Geometry check sheet. Reference: drawing and pictorial views, mm from the part's lowest x, y, z. Round coordinates to 2 decimals unless told otherwise and drop trailing zeros. Loops run counter-clockwise (first coordinate to the right, second up) from the corner with the lowest first, then second, coordinate; pieces in that order, holes last. Notation, with made-up numbers: (-33.75, -22) -> (-19.75, -22) arc R22 cw to (-19.75, -13) -> close; hole circle Ø10 at (86.5, -14). An arc over 180 degrees is marked (long way). Write item = value, one per line.
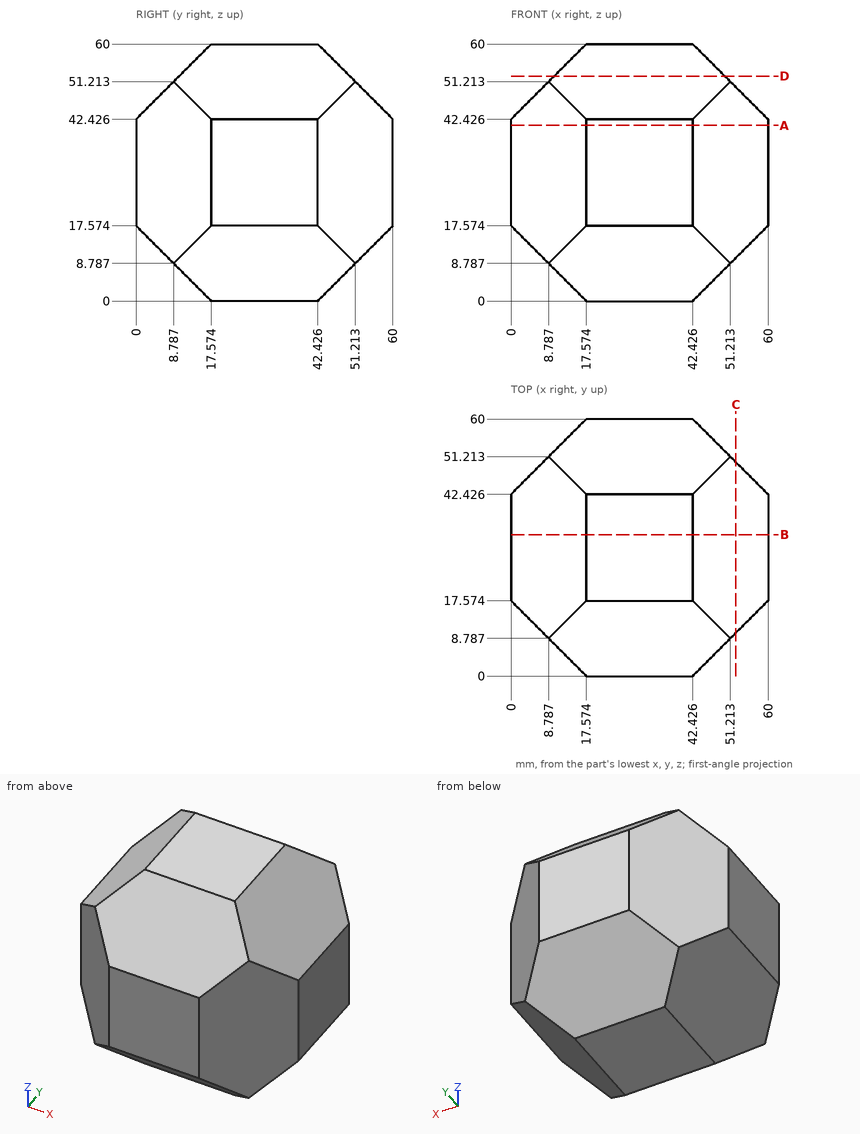
(1) Material ranges on probe 1 along Z at (x, y) = (42.5, 3) (1 decimal); probe 2 along Z at (x, y) = (10.5, 16) (1 decimal); probe 3 along Y at (x, z) = (37, 13.5) (1 decimal), recorded low to high. Write a range as from..to.
Filled sheet:
probe_1 = 14.6..45.4
probe_2 = 7.1..52.9
probe_3 = 4.1..55.9
(2) Sectioned sample at C-C, the plane x = 52.5. Record the cut outline in (y, z).
Filled sheet:
outline = (10.07, 10.07) -> (49.93, 10.07) -> (49.93, 49.93) -> (10.07, 49.93) -> close
(3) Go/stop test with flat-tipped pins: pin 1 Ø1.5 at (x, z) = (51, 35) entering from -Y (1 decimal); pin 2 Ø3 at (x, y) = (46.5, 29.5) entering from -Z (1 decimal); pin 3 Ø12 at (y, z) = (27.5, 13) entering from -X; pin 4 Ø8 at (y, z) = (53, 18.5) entering from +X (1 decimal). Record where each tip stops, or that it passes through.
Filled sheet:
pin_1 = 7.8
pin_2 = 2.6
pin_3 = 0
pin_4 = 53.4
(4) Sectioned sample at A-A, the plane z = 41. Record the cut outline in (x, y), and give its area (3 significant figures).
Filled sheet:
outline = (0, 17.57) -> (17.57, 0) -> (42.43, 0) -> (60, 17.57) -> (60, 42.43) -> (42.43, 60) -> (17.57, 60) -> (0, 42.43) -> close
area = 2,980 mm2
